```python
from build123d import *

# Parameters (mm, degrees)
CYLINDER001_R     = 1.6
CYLINDER001_DEPTH = 10
CYLINDER_R        = 1.6
CYLINDER_DEPTH    = 10
CYLINDER002_R     = 1.6
CYLINDER002_DEPTH = 10
CYLINDER003_R     = 1.6
CYLINDER003_DEPTH = 10
CYLINDER004_R     = 1.6
CYLINDER004_DEPTH = 10
BOX_W             = 50
BOX_H             = 10
BOX_DEPTH         = 3


with BuildPart() as cylinder001:
    # Cylinder001 → Cylinder001 (new body)
    with BuildSketch(Plane(origin=(15, 5, -3), x_dir=(1, 0, 0), z_dir=(0, 0, 1))):
        Circle(CYLINDER001_R)
    extrude(amount=CYLINDER001_DEPTH)


with BuildPart() as cylinder:
    # Cylinder → Cylinder (new body)
    with BuildSketch(Plane(origin=(5, 5, -3), x_dir=(1, 0, 0), z_dir=(0, 0, 1))):
        Circle(CYLINDER_R)
    extrude(amount=CYLINDER_DEPTH)


with BuildPart() as cylinder002:
    # Cylinder002 → Cylinder002 (new body)
    with BuildSketch(Plane(origin=(25, 5, -3), x_dir=(1, 0, 0), z_dir=(0, 0, 1))):
        Circle(CYLINDER002_R)
    extrude(amount=CYLINDER002_DEPTH)


with BuildPart() as cylinder003:
    # Cylinder003 → Cylinder003 (new body)
    with BuildSketch(Plane(origin=(35, 5, -3), x_dir=(1, 0, 0), z_dir=(0, 0, 1))):
        Circle(CYLINDER003_R)
    extrude(amount=CYLINDER003_DEPTH)


with BuildPart() as fusion:
    # Cylinder004 → Cylinder004 (new body)
    with BuildSketch(Plane(origin=(45, 5, -3), x_dir=(1, 0, 0), z_dir=(0, 0, 1))):
        Circle(CYLINDER004_R)
    extrude(amount=CYLINDER004_DEPTH)

    # Fusion: union Cylinder001, Cylinder, Cylinder002, Cylinder003
    add(cylinder001.part)
    add(cylinder.part)
    add(cylinder002.part)
    add(cylinder003.part)


with BuildPart() as cut:
    # Box → Box (new body)
    with BuildSketch(Plane.XY):
        with Locations((25, 5)):
            Rectangle(BOX_W, BOX_H)
    extrude(amount=BOX_DEPTH)

    # Cut: cut Fusion
    add(fusion.part, mode=Mode.SUBTRACT)


solid = cut.part
```
The listing builds one solid part. Answer for the finished solid, in the listing's coordinates (mm). Give positions to 0.01 mm unless a question says otherwise; leave off trailing zeros. Write each loop counter-clockwise with the first axis right and the second up, starting at its lowest first coordinate (ties: lowest second). Pieces come first, ordered by that corner, then holes. Notation, with made-up numbers: (33, -37) - (43, -37) arc R7 cw to (43, -33) - close; hole circle Ø1 at (8.25, -15.5). An arc over 180 degrees is marked (long way). Use one line per item in the form item = value. Start each with the question number.
1) Find section A-A on y = 5. Determine the outline of the cut face in (x, z).
2) A flat-ended cylindrical pin translates along its axis: pin 1 Ø4 at (x, y) = (15, 5) entering from -Z. Find the tip coordinate at first contact, or state that the pin passes through.
3) Consider line 1 along X through (y, z) = (5, 0.85); line 2 along X through (y, z) = (5.5, 0.8); line 3 along Y through (x, z) = (45, 1.15). Determine where each line is inside the solid, lowest interval first. Write a range as from..to.
4) Find section B-B on x = 25. Determine the outline of the cut face in (y, z), plus the area to 3 significant figures.
5) Find section C-C on z = 2.05. Determine the outline of the cut face in (x, y).
6) The mould has two halves that part along X. Classify faces 1 (the face through (0, 5, 1)), 2 (the face through (25, 7, 0)), 3 (the face through (4.65, 3.44, 1.48)): pulls with the +X half, pulls with the -X half, needs draft (parallel to the pull), parting line crosses it, or undercut.
Geometry results:
q1.outline = (0, 0) - (3.4, 0) - (3.4, 3) - (0, 3) - close; (6.6, 0) - (13.4, 0) - (13.4, 3) - (6.6, 3) - close; (16.6, 0) - (23.4, 0) - (23.4, 3) - (16.6, 3) - close; (26.6, 0) - (33.4, 0) - (33.4, 3) - (26.6, 3) - close; (36.6, 0) - (43.4, 0) - (43.4, 3) - (36.6, 3) - close; (46.6, 0) - (50, 0) - (50, 3) - (46.6, 3) - close
q2.pin_1 = 0
q3.line_1 = 0..3.4, 6.6..13.4, 16.6..23.4, 26.6..33.4, 36.6..43.4, 46.6..50
q3.line_2 = 0..3.48, 6.52..13.48, 16.52..23.48, 26.52..33.48, 36.52..43.48, 46.52..50
q3.line_3 = 0..3.4, 6.6..10
q4.outline = (0, 0) - (3.4, 0) - (3.4, 3) - (0, 3) - close; (6.6, 0) - (10, 0) - (10, 3) - (6.6, 3) - close
q4.area = 20.4 mm2
q5.outline = (0, 0) - (50, 0) - (50, 10) - (0, 10) - close; hole circle Ø3.2 at (5, 5); hole circle Ø3.2 at (15, 5); hole circle Ø3.2 at (25, 5); hole circle Ø3.2 at (35, 5); hole circle Ø3.2 at (45, 5)
q6.face_1 = pulls with the -X half
q6.face_2 = needs draft
q6.face_3 = undercut
